from build123d import *

# Parameters (mm, degrees)
SKETCH1_W           = 33
SKETCH1_H           = 33.83
BOSS_EXTRUDE1_DEPTH = 5
SKETCH2_W           = 29
SKETCH2_H           = 29.83
CUT_EXTRUDE1_DEPTH  = 1.5
SKETCH3_R           = 1.5
CUT_EXTRUDE3_DEPTH  = 31
CUT_EXTRUDE4_DEPTH  = 2
FILLET1_R           = 2
SKETCH5_W           = 11.644842875
SKETCH5_H           = 2.596903013
CUT_EXTRUDE5_DEPTH  = 2
CUT_EXTRUDE9_DEPTH  = 10
FILLET5_R           = 1
FILLET6_R           = 1


with BuildPart() as part:
    # Sketch1 → Boss-Extrude1 (new body)
    with BuildSketch(Plane(origin=(0, 0, 0), x_dir=(1, 0, 0), z_dir=(0, 1, 0))):
        Rectangle(SKETCH1_W, SKETCH1_H)
    extrude(amount=-BOSS_EXTRUDE1_DEPTH)

    # Sketch2 → Cut-Extrude1 (cut)
    with BuildSketch(Plane(origin=(0, 0, 0), x_dir=(1, 0, 0), z_dir=(0, 1, 0))):
        Rectangle(SKETCH2_W, SKETCH2_H)
    extrude(amount=-CUT_EXTRUDE1_DEPTH, mode=Mode.SUBTRACT)

    # Sketch3 → Cut-Extrude3 (cut)
    with BuildSketch(Plane(origin=(0, 0, 0), x_dir=(1, 0, 0), z_dir=(0, 1, 0))):
        with Locations(Location((0.5, 7.915, 0), (0, 0, 270))):
            Circle(SKETCH3_R)
        with Locations(Location((0.5, -9.885, 0), (0, 0, 270))):
            Circle(SKETCH3_R)
    extrude(amount=-CUT_EXTRUDE3_DEPTH, mode=Mode.SUBTRACT)

    # Sketch4 → Cut-Extrude4 (cut)
    with BuildSketch(Plane.XZ.offset(5)):
        with BuildLine():
            Line((-4.5, 9.885), (-4.5, -7.915))
            ThreePointArc((-4.5, -7.915), (0.5, -12.915), (5.5, -7.915))
            Line((5.5, -7.915), (5.5, 9.885))
            ThreePointArc((5.5, 9.885), (0.5, 14.885), (-4.5, 9.885))
        make_face()
    extrude(amount=-CUT_EXTRUDE4_DEPTH, mode=Mode.SUBTRACT)

    # Fillet1
    fillet1_edges = [part.edges().sort_by_distance(p)[0] for p in [
        (14.5, -0.75, 14.915),
        (-14.5, -0.75, 14.915),
        (-14.5, -0.75, -14.915),
        (14.5, -0.75, -14.915),
        (16.5, -2.5, 16.915),
        (-16.5, -2.5, 16.915),
        (-16.5, -2.5, -16.915),
        (16.5, -2.5, -16.915),
    ]]
    fillet(fillet1_edges, radius=FILLET1_R)

    # Sketch5 → Cut-Extrude5 (cut)
    with BuildSketch(Plane.XZ.offset(5)):
        with Locations((0.473449804, 8.503582245)):
            Rectangle(SKETCH5_W, SKETCH5_H)
    extrude(amount=-CUT_EXTRUDE5_DEPTH, mode=Mode.SUBTRACT)

    # Sketch7 → Cut-Extrude9 (cut)
    with BuildSketch(Plane.XY.offset(16.915)):
        Polygon((0.5, 0), (-6.67, 0), (-6.67, -1.5), (7.67, -1.5), (7.67, 0), align=None)
    extrude(amount=-CUT_EXTRUDE9_DEPTH, mode=Mode.SUBTRACT)

    # Fillet5
    fillet5_edges = [part.edges().sort_by_distance(p)[0] for p in [
        (-6.67, -1.5, 15.915),
    ]]
    fillet(fillet5_edges, radius=FILLET5_R)

    # Fillet6
    fillet6_edges = [part.edges().sort_by_distance(p)[0] for p in [
        (7.67, -1.5, 15.915),
    ]]
    fillet(fillet6_edges, radius=FILLET6_R)


solid = part.part
Could you check a few things on this model? Use its own coordinates, in mm. A direction names the side the tool comes from. Give positions to 0.01 mm unless a question says otherwise; leave off trailing zeros. Order: outer loops, then holes, each group sorted by start corner. A loop starts at its lowest first (then second) coordinate and runs counter-clockwise, first axis right, second up.
1. I need wall thicknesses on L1, parallel to X at y = -0.8, z = -8.5; L2, parallel to X at y = -3.85, z = -1; L3, parallel to Z at x = 10, y = -0.25 (3 decimals). Which ranges of each line are inside material? Lowest first, please.
2. We'd pull the mould along X, two halves only. Please class faces 1 (the flat face through (0, -3, 16.915)), 2 (the flat face through (0, -1, -14.915)), 3 (the cylindrical face through (-15.93, -2.535, -16.314)), 4 (the flat face through (-14.5, -1, 0)): pulls with the +X half, pulls with the -X half, needs draft (parallel to the pull), parting line crosses it, or undercut.
3. Suppose I cut it at A-A (y = -2.35). List the corners of the cut face in (x, z) for me (3 decimals).
4. Will this pin go through, and if not, where does the flat tip stop? P1, Ø2, axis at x = -11.5, z = 10.5, coming from the +Y side.
5. For faces 5 (the flat face through (-0.1, 0, -15.1)), 6 (the cylindrical face through (-6.385, -1.199, 15.901)), 7 (the flat face through (10, -1, 14.915)), 8 (the cylindrical face through (15.899, -2.535, 16.345)), 9 (the cylindrical face through (0.61, -4.014, 14.884)), which set-ups out of +Z, -Z, +X, -X, +Y, -Y let a thin tool reach every point of the face, with its end or its side?
6. Suppose I cut it at D-D (x = 11.5). List the corners of the cut face in (y, z) for me (3 decimals), plus the area to 3 significant figures.
7. Suppose I cut it at C-C (z = 1.5). List the corners of the cut face in (x, y) for me.
8. Suppose I cut it at B-B (x = 0.5). List the corners of the cut face in (y, z) for me (3 decimals).
Solved:
1. L1: x = -16.5 to -14.5, 14.5 to 16.5
1. L2: x = -16.5 to -4.5, 5.5 to 16.5
1. L3: z = -16.915 to -14.915, 14.915 to 16.915
2. face 1: needs draft
2. face 2: undercut
2. face 3: pulls with the -X half
2. face 4: undercut
3. outline: (-16.5, -14.915) arc R2 ccw to (-14.5, -16.915) - (14.5, -16.915) arc R2 ccw to (16.5, -14.915) - (16.5, 14.915) arc R2 ccw to (14.5, 16.915) - (-14.5, 16.915) arc R2 ccw to (-16.5, 14.915) - close; hole circle Ø3 at (0.5, -7.915); hole circle Ø3 at (0.5, 9.885)
4. P1: stops at y = -1.5
5. face 5: +Z, -Z, +X, -X, +Y
5. face 6: +Z, +Y
5. face 7: +Y
5. face 8: +Z, +X, +Y, -Y
5. face 9: -Y
6. outline: (-5, -16.915) - (0, -16.915) - (0, -14.915) - (-1.5, -14.915) - (-1.5, 14.915) - (0, 14.915) - (0, 16.915) - (-5, 16.915) - close
6. area: 124 mm2
7. outline: (-16.5, -5) - (-4.5, -5) - (-4.5, -3) - (5.5, -3) - (5.5, -5) - (16.5, -5) - (16.5, 0) - (14.5, 0) - (14.5, -1.5) - (-14.5, -1.5) - (-14.5, 0) - (-16.5, 0) - close
8. outline: (-5, -16.915) - (0, -16.915) - (0, -14.915) - (-1.5, -14.915) - (-1.5, -9.415) - (-3, -9.415) - (-3, -12.915) - (-5, -12.915) - close; (-5, 14.885) - (-3, 14.885) - (-3, 11.385) - (-1.5, 11.385) - (-1.5, 16.915) - (-5, 16.915) - close; (-3, -6.415) - (-1.5, -6.415) - (-1.5, 8.385) - (-3, 8.385) - close
